```python
from build123d import *

# Parameters (mm, degrees)
F0_W     = 787.4
F0_H     = 177.8
F1_DEPTH = 19.05
F4_D     = 12.7
F5_D     = 9.525
F7_DEPTH = 6.35
F8_D     = 12.7


with BuildPart() as f1:
    # F0 (on Right) → F1 (new body)
    with BuildSketch(Plane.YZ):
        with Locations((29.7667551786, 66.8366326568)):
            Rectangle(F0_W, F0_H)
    extrude(amount=F1_DEPTH)

    # F4 (through all)
    with Locations(Plane.YZ.offset(19.05)):
        with Locations((156.7667551786, 47.7866326568), (258.3667551786, 47.7866326568), (359.9667551786, 47.7866326568)):
            Hole(F4_D / 2)

    # F5 (through all)
    with Locations(Plane.XY.offset(155.7366326568)):
        with Locations((6.35, -173.4332448214), (6.35, -249.6332448214), (6.35, -325.8332448214)):
            Hole(F5_D / 2)

    # F6 (on face) → F7 (join, symmetric)
    with BuildSketch(Plane.YZ.offset(19.05)):
        with BuildLine():
            Line((423.4667551786, 111.2866326568), (423.4667551786, 133.5116326568))
            Line((423.4667551786, 133.5116326568), (0, 133.5116326568))
            Line((0, 133.5116326568), (0, 111.2866326568))
            Line((0, 111.2866326568), (151.2674938645, 111.2866326568))
            ThreePointArc((151.2674938645, 111.2866326568), (155.1232542422, 120.5952616538), (163.1167551786, 114.4616326568))
            Line((163.1167551786, 114.4616326568), (252.0167551786, 114.4616326568))
            ThreePointArc((252.0167551786, 114.4616326568), (258.3667551786, 120.8116326568), (264.7167551786, 114.4616326568))
            Line((264.7167551786, 114.4616326568), (353.6167551786, 114.4616326568))
            ThreePointArc((353.6167551786, 114.4616326568), (359.9667551786, 120.8116326568), (366.3167551786, 114.4616326568))
            ThreePointArc((366.3167551786, 114.4616326568), (366.1003841755, 112.8181317204), (365.4660164926, 111.2866326568))
            Line((365.4660164926, 111.2866326568), (423.4667551786, 111.2866326568))
        make_face()
    extrude(amount=F7_DEPTH, both=True)

    # F8 (through all)
    with Locations(Plane.YZ.offset(19.05)):
        with Locations((359.9667551786, 114.4616326568), (258.3667551786, 114.4616326568), (156.7667551786, 114.4616326568)):
            Hole(F8_D / 2)


solid = f1.part
```
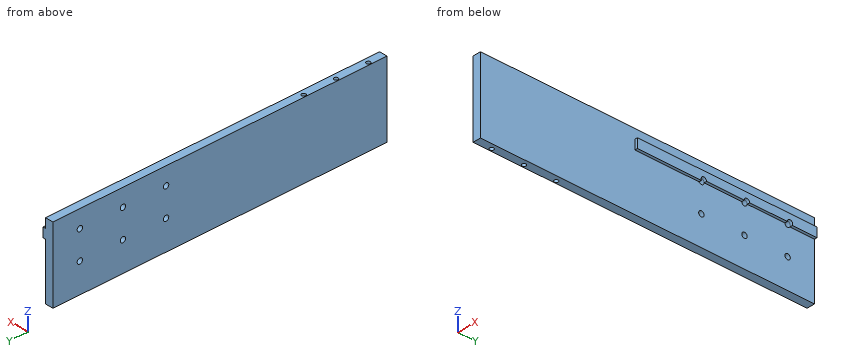
The model under review builds one solid part; all positions refer to its coordinate system, in mm. Give positions to 0.01 mm unless a question says otherwise; leave off trailing zeros. Write each loop counter-clockwise with the first axis right and the second up, starting at its lowest first coordinate (ties: lowest second). Pieces come first, ordered by that corner, then holes. Notation, with made-up numbers: (-27, -19) -> (9, -19) arc R14 ccw to (9, 1) -> close; hole circle Ø10 at (19, 12.5). An arc over 180 degrees is marked (long way). Put each result on its own line as item: value.
(1) We need section B-B, the plane y = 314. Give the boundary of the cut face in (x, z).
Results are:
outline: (0, -22.06) -> (19.05, -22.06) -> (19.05, 114.46) -> (25.4, 114.46) -> (25.4, 133.51) -> (19.05, 133.51) -> (19.05, 155.74) -> (0, 155.74) -> close
(2) For pin 1 Ø2 at (y, z) = (-32, 29.5) entering from +X; pin 2 Ø1.9 at (x, z) = (23.5, 125) entering from -Y; pin 3 Ø1.9 at (x, y) = (22, 320.5) entering from -Z, all flat-tipped, find the tip position at first contact; note any pin that passes through.
Results are:
pin 1: x = 19.05
pin 2: y = 0
pin 3: z = 114.46
(3) We need section D-D, the plane y = 78. Give the boundary of the cut face in (x, z).
Results are:
outline: (0, -22.06) -> (19.05, -22.06) -> (19.05, 111.29) -> (25.4, 111.29) -> (25.4, 133.51) -> (19.05, 133.51) -> (19.05, 155.74) -> (0, 155.74) -> close
(4) To check wall thickness, follow probe 1 along Y at (x, z) = (6.35, 19); probe 2 along Y at (x, z) = (3.75, 26); probe 3 along X at (y, z) = (-332, 78.5). State the ranges of each line that lie inside material, in increasing order. Write a range as from..to.
Results are:
probe 1: -363.93..-330.6, -321.07..-254.4, -244.87..-178.2, -168.67..423.47
probe 2: -363.93..-329.82, -321.84..-253.62, -245.64..-177.42, -169.44..423.47
probe 3: 0..19.05
(5) We need section A-A, the plane x = 6.35. State how many separate pieces and enclosed holes the cut face has, and give its area (3 significant figures).
Results are:
separate pieces: 4
enclosed holes: 6
area: 134,000 mm²
